from build123d import *

# Parameters (mm, degrees)
F0_W      = 469.9
F0_H      = 463.55
F1_DEPTH  = 19.05
F3_D      = 15.0114
F3_DEPTH  = 14.224
F3_TIP    = 4.5098795482
F5_D      = 8.001
F5_DEPTH  = 25.4
F5_TIP    = 2.4037429064
F7_D      = 8.001
F7_DEPTH  = 25.4
F7_TIP    = 2.4037429064
F9_D      = 8.001
F9_DEPTH  = 25.4
F9_TIP    = 2.4037429064
F11_D     = 8.001
F11_DEPTH = 19.05
F11_TIP   = 2.4037429064


with BuildPart() as f1:
    # F0 (on Top) → F1 (new body)
    with BuildSketch(Plane.XY):
        Rectangle(F0_W, F0_H)
    extrude(amount=F1_DEPTH)

    # F3
    with Locations(Plane(origin=(0, 0, 0), x_dir=(1, 0, 0), z_dir=(0, 0, -1))):
        with Locations((-211.074, 180.975), (-211.074, 0), (-211.074, -180.975), (-184.15, -207.899), (0, -207.899), (184.15, -207.899), (211.074, -180.975), (211.074, 0), (211.074, 180.975)):
            Hole(F3_D / 2, depth=F3_DEPTH)
            with Locations((0, 0, -(F3_DEPTH + F3_TIP / 2))):  # 118° drill point
                Cone(0, F3_D / 2, F3_TIP, mode=Mode.SUBTRACT)

    # F5
    with Locations(Plane.YZ.offset(234.95)):
        with Locations((-180.975, 9.525), (0, 9.525), (180.975, 9.525)):
            Hole(F5_D / 2, depth=F5_DEPTH)
            with Locations((0, 0, -(F5_DEPTH + F5_TIP / 2))):  # 118° drill point
                Cone(0, F5_D / 2, F5_TIP, mode=Mode.SUBTRACT)

    # F7
    with Locations(Plane(origin=(0, 231.775, 0), x_dir=(-1, 0, 0), z_dir=(0, 1, 0))):
        with Locations((-184.15, 9.525), (0, 9.525), (184.15, 9.525)):
            Hole(F7_D / 2, depth=F7_DEPTH)
            with Locations((0, 0, -(F7_DEPTH + F7_TIP / 2))):  # 118° drill point
                Cone(0, F7_D / 2, F7_TIP, mode=Mode.SUBTRACT)

    # F9
    with Locations(Plane(origin=(-234.95, 0, 0), x_dir=(0, -1, 0), z_dir=(-1, 0, 0))):
        with Locations((-180.975, 9.525), (0, 9.525), (180.975, 9.525)):
            Hole(F9_D / 2, depth=F9_DEPTH)
            with Locations((0, 0, -(F9_DEPTH + F9_TIP / 2))):  # 118° drill point
                Cone(0, F9_D / 2, F9_TIP, mode=Mode.SUBTRACT)

    # F11
    with Locations(Plane.XY.offset(19.05)):
        with Locations((-152.4, 180.975), (152.4, 180.975), (152.4, -174.625), (-152.4, -174.625)):
            Hole(F11_D / 2, depth=F11_DEPTH)
            with Locations((0, 0, -(F11_DEPTH + F11_TIP / 2))):  # 118° drill point
                Cone(0, F11_D / 2, F11_TIP, mode=Mode.SUBTRACT)


solid = f1.part
The listing builds one solid part. Answer for the finished solid, in the listing's coordinates (mm). A direction names the side the tool comes from. Give positions to 0.01 mm unless a question says otherwise; leave off trailing zeros. Answer as a JSON object with one key per item and string values.
1. For a pull along X with two mould halves and no side action, classify faces 1 (the flat face through (-234.95, -3, 14)), 2 (the flat face through (-3, -231.775, 9)), 3 (the cylindrical face through (-203.576, -0.33, 7.212)) as pulls with the +X half, pulls with the -X half, needs draft (parallel to the pull), parting line crosses it, or undercut.
Determined:
{"face 1": "pulls with the -X half", "face 2": "needs draft", "face 3": "undercut"}
2. For faces 4 (the flat face through (-3, 3, 0)), 5 (the cylindrical face through (204.14, -178.1, 7.21)), determine the directions among +Z, -Z, +X, -X, +Y, -Y from which every point of the face is accessible in a straight line to the end or side of a thin tool.
Determined:
{"face 4": "-Z, +X, -X, +Y, -Y", "face 5": "-Z"}
3. Flat-ended cylindrical pins translate along their axes: pin 1 Ø6.5 at (x, z) = (0, 9.525) entering from +Y; pin 2 Ø12 at (x, y) = (0, 207.899) entering from -Z; pin 3 Ø9 at (x, y) = (211.074, 180.975) entering from -Z. Find the tip coordinate at first contact, or state that the pin passes through.
Determined:
{"pin 1": "y = 201.13", "pin 2": "z = 15.13", "pin 3": "z = 16.03"}
4. Find the intervals of material crossed by L1, parallel to Y at x = 182.5, z = 10.5 (3 decimals), in increasing order. Write a range as [from, to].
Determined:
{"L1": "[-231.775, 200.577]"}
